```python
from build123d import *

# Parameters (mm, degrees)
SKETCH_6_R          = 4.5
EXTRUDE_4_DEPTH     = 3
SKETCH_7_R          = 3.15
CUT_EXTRUDE_4_DEPTH = 2
SKETCH_8_R          = 4
EXTRUDE_5_DEPTH     = 2
EXTRUDE_7_DEPTH     = 2
EXTRUDE_8_REACH     = 10
SKETCH_11_R         = 1.65
CUT_EXTRUDE_6_DEPTH = 2
CUT_EXTRUDE_7_REACH = 9
FILLET_1_R          = 0.3
FILLET_2_R          = 0.3
FILLET_3_R          = 0.3


with BuildPart() as part:
    # Sketch 6 → Extrude 4 (new body)
    with BuildSketch(Plane(origin=(0, 0, 0), x_dir=(1, 0, 0), z_dir=(0, 1, 0))):
        Circle(SKETCH_6_R)
    extrude(amount=-EXTRUDE_4_DEPTH)

    # Sketch 7 → Cut-Extrude 4 (cut)
    with BuildSketch(Plane(origin=(0, 0, 0), x_dir=(1, 0, 0), z_dir=(0, 1, 0))):
        Circle(SKETCH_7_R)
    extrude(amount=-CUT_EXTRUDE_4_DEPTH, mode=Mode.SUBTRACT)

    # Sketch 15 → Cut-Revolve 2 (revolve, cut)
    with BuildSketch(Plane(origin=(0, 0, 0), x_dir=(0, 0, -1), z_dir=(1, 0, 0))):
        Polygon((4.5, -3), (4.5, -2), (3.5, -3), align=None)
    revolve(axis=Axis((0, 0, 0), (0, -1, 0)), mode=Mode.SUBTRACT)



with BuildPart() as body_2:
    # Sketch 8 → Extrude 5 (new body)
    with BuildSketch(Plane(origin=(-0.5, 0, 0), x_dir=(0, 0, -1), z_dir=(1, 0, 0))):
        with Locations((-9, 2.5)):
            Circle(SKETCH_8_R)
    extrude(amount=-EXTRUDE_5_DEPTH)


with BuildPart() as part_1:
    add(part.part)

    add(body_2.part)  # Extrude 7 merges body 2
    # Sketch 9 → Extrude 7 (add)
    with BuildSketch(Plane(origin=(-0.5, 0, 0), x_dir=(0, 0, -1), z_dir=(1, 0, 0))):
        Polygon((-4.5, -3), (-10.133083988, -1.336159626), (-5.152908316, 3.69564436), (-3.5, 0), (-3.5, -3), (-3.52896076, -3), align=None)
    extrude(amount=-EXTRUDE_7_DEPTH)

    # Sketch 16 → Extrude 8 (add, up to next)
    with BuildSketch(Plane(origin=(0, 0, 3.5), x_dir=(-1, 0, 0), z_dir=(0, 0, -1)), mode=Mode.PRIVATE) as extrude_8_sk1:
        Polygon((2.5, -3), (2.5, -2.198837366), (0.5, -2.955716811), (0.5, -3), align=None)
    extrude_8_tool1 = extrude(extrude_8_sk1.sketch, amount=EXTRUDE_8_REACH, mode=Mode.PRIVATE) - part_1.part
    add(extrude_8_tool1.solids().sort_by_distance((-1.798414, -2.732173, 3.5))[0])

    # Sketch 11 → Cut-Extrude 6 (cut)
    with BuildSketch(Plane(origin=(-0.5, 0, 0), x_dir=(0, 0, -1), z_dir=(1, 0, 0))):
        with Locations((-9, 2.5)):
            Circle(SKETCH_11_R)
    extrude(amount=-CUT_EXTRUDE_6_DEPTH, mode=Mode.SUBTRACT)

    # Sketch 12 → Cut-Extrude 7 (cut, up to next)
    with BuildSketch(Plane.ZY.offset(2.5), mode=Mode.PRIVATE) as cut_extrude_7_sk1:
        Polygon((3.5, 0), (3.741657387, 0), (5.175729917, 3.672586172), (5.152908316, 3.69564436), align=None)
    cut_extrude_7_tool1 = extrude(cut_extrude_7_sk1.sketch, amount=-CUT_EXTRUDE_7_REACH, mode=Mode.PRIVATE) & part_1.part
    add(cut_extrude_7_tool1.solids().sort_by_distance((-2.5, 1.373556, 4.196165))[0], mode=Mode.SUBTRACT)

    # Fillet 1
    fillet_1_edges = [part_1.edges().sort_by_distance(p)[0] for p in [
        (-3.15, 0, 0),
    ]]
    fillet(fillet_1_edges, radius=FILLET_1_R)

    # Fillet 2
    fillet_2_edges = [part_1.edges().sort_by_distance(p)[0] for p in [
        (-0.5, 2.5, 10.65),
    ]]
    fillet(fillet_2_edges, radius=FILLET_2_R)

    # Fillet 3
    fillet_3_edges = [part_1.edges().sort_by_distance(p)[0] for p in [
        (-2.5, 2.5, 10.65),
    ]]
    fillet(fillet_3_edges, radius=FILLET_3_R)


solid = part_1.part
```
Work out the finished part from the listing and answer in its coordinate system (mm). A direction names the side the tool comes from. Coordinates: 2 decimals unless noted, no trailing zeros. Write each loop counter-clockwise with the first axis right and the second up, starting at its lowest first coordinate (ties: lowest second). Pieces come first, ordered by that corner, then holes. Notation, with made-up numbers: (66.25, -35.75) - (115.25, -35.75) arc R14 cw to (115.25, -8.75) - close; hole circle Ø10 at (-36.5, 12.25). An arc over 180 degrees is marked (long way). Answer as a JSON object with one key per item and string values.
Q1. Find section B-B (y = 2.5). Write down the section's boundary in (x, z).
Results list:
{"outline": "(-2.5, 4.72) - (-0.5, 4.72) - (-0.5, 7.05) arc R0.3 ccw to (-0.8, 7.35) - (-2.2, 7.35) arc R0.3 ccw to (-2.5, 7.05) - close; (-2.5, 10.95) arc R0.3 ccw to (-2.2, 10.65) - (-0.8, 10.65) arc R0.3 ccw to (-0.5, 10.95) - (-0.5, 13) - (-2.5, 13) - close"}
Q2. Which of the six approach directions +Z, -Z, +X, -X, +Y, -Y give full straight-line access (tool end or side, diameter ignored) to faces 1 (the cylindrical face through (1.714, -0.986, -4.161)), 2 (the cylindrical face through (-2.5, -1.138, 1.917))?
Results list:
{"face 1": "+Y, -Y", "face 2": "+Y"}
Q3. Given pin 1 Ø3 at (y, z) = (3, 9.5) entering from -X; pin 2 Ø4 at (x, y) = (-0.5, -2) entering from +Z; pin 3 Ø5 at (x, y) = (3, 0.5) entering from +Z, each flat-ended and moving along its own axis, determine where each tip first touches the part or whether it passes through.
Results list:
{"pin 1": "stops at x = -2.5", "pin 2": "stops at z = 12.12", "pin 3": "stops at z = 4.47"}
Q4. Find section D-D (z = 0). Write down the section's boundary in (x, y), plus the area to 3 significant figures.
Results list:
{"outline": "(-4.5, -2) - (-3.5, -3) - (3.5, -3) - (4.5, -2) - (4.5, 0) - (3.45, 0) arc R0.3 ccw to (3.15, -0.3) - (3.15, -2) - (-3.15, -2) - (-3.15, -0.3) arc R0.3 ccw to (-3.45, 0) - (-4.5, 0) - close", "area": "13.4 mm^2"}
Q5. Consider L1, parallel to Y at x = 1.5, z = -1.25; L2, parallel to X at y = -1.55, z = 0; L3, parallel to Z at x = -1, y = 3. Determine where each line is inside the solid, lowest interval first. Write a range as from..to.
Results list:
{"L1": "y = -3..-2", "L2": "x = -4.5..-3.15, 3.15..4.5", "L3": "z = 4.91..7.43, 10.57..12.97"}
Q6. Find section C-C (x = 0). Write down the section's boundary in (y, z).
Results list:
{"outline": "(-3, -3.5) - (-2, -4.5) - (0, -4.5) - (0, -3.45) arc R0.3 ccw to (-0.3, -3.15) - (-2, -3.15) - (-2, 3.15) - (-0.3, 3.15) arc R0.3 ccw to (0, 3.45) - (0, 4.5) - (-2, 4.5) - (-3, 3.5) - close"}
Q7. Find section A-A (z = 9). Write down the section's boundary in (x, y), plus the area to 3 significant figures.
Results list:
{"outline": "(-2.5, -1.67) - (-0.5, -1.67) - (-0.5, 0.55) arc R0.3 ccw to (-0.8, 0.85) - (-2.2, 0.85) arc R0.3 ccw to (-2.5, 0.55) - close; (-2.5, 4.45) arc R0.3 ccw to (-2.2, 4.15) - (-0.8, 4.15) arc R0.3 ccw to (-0.5, 4.45) - (-0.5, 6.5) - (-2.5, 6.5) - close", "area": "9.66 mm^2"}
Q8. For a pull along X with two mould halves and no side action, classify faces 3 (the flat face through (-2.5, 0.6, 7.8)), 4 (the flat face through (0, -3, 1)), 5 (the flat face through (0, -2, 0)) as pulls with the +X half, pulls with the -X half, needs draft (parallel to the pull), parting line crosses it, or undercut.
Results list:
{"face 3": "pulls with the -X half", "face 4": "needs draft", "face 5": "undercut"}
